from build123d import *

# Parameters (mm, degrees)
BOSS_EXTRUDE1_DEPTH = 29.765625
SKETCH3_R           = 29.464
OLEOPIST_DEPTH      = 397.764
SKETCH5_R           = 32.004
REFMAXOLEO_DEPTH    = 2.54
SKETCH7_R           = 9.525
BOSS_EXTRUDE4_DEPTH = 15.875


with BuildPart() as part:
    # Sketch1 → Boss-Extrude1 (new, symmetric)
    with BuildSketch(Plane.XY):
        with BuildLine():
            Line((-114.3, -150.1775), (-114.3, 150.1775))
            ThreePointArc((-114.3, 150.1775), (-99.421024484, 186.098524484), (-63.5, 200.9775))
            Line((-63.5, 200.9775), (15.875, 200.9775))
            Line((15.875, 200.9775), (15.875, 251.7775))
            Line((15.875, 251.7775), (-63.5, 251.7775))
            ThreePointArc((-63.5, 251.7775), (-135.342048969, 222.019548969), (-165.1, 150.1775))
            Line((-165.1, 150.1775), (-165.1, -150.1775))
            Line((-165.1, -150.1775), (-114.3, -150.1775))
        make_face()
    extrude(amount=BOSS_EXTRUDE1_DEPTH, both=True)

    # Sketch2 → Revolve1 (revolve)
    with BuildSketch(Plane.XZ.offset(150.1775)):
        Polygon((-165.1, 0), (-114.3, 0), (-50.8, 0), (-50.8, 81.915), (-76.2, 81.915), (-76.2, 31.75), (-114.3, 31.75), (-114.3, 37.20703125), (-165.1, 37.20703125), align=None)
    revolve(axis=Axis((-165.1, -150.1775, 0), (1, 0, 0)))

    # Sketch3 → OleoPist (add)
    with BuildSketch(Plane.XZ.offset(-200.9775)):
        with Locations(Location((15.875, 0, 0), (0, 0, 237.398482094))):
            Circle(SKETCH3_R)
    extrude(amount=-OLEOPIST_DEPTH)

    # Sketch5 → RefMaxOleo (add)
    with BuildSketch(Plane(origin=(0, 340.6775, 0), x_dir=(1, 0, 0), z_dir=(0, 1, 0))):
        with Locations(Location((15.875, 0, 0), (0, 0, 180))):
            Circle(SKETCH5_R)
    extrude(amount=-REFMAXOLEO_DEPTH)

    # Sketch7 → Boss-Extrude4 (add, symmetric)
    with BuildSketch(Plane(origin=(15.875, -150.1775, 0), x_dir=(0, 0, -1), z_dir=(1, 0, 0))):
        with BuildLine():
            Line((16.764, 488.315), (59.880363403, 435.864541166))
            ThreePointArc((59.880363403, 435.864541166), (65.58043358, 421.731246842), (62.165446707, 406.879355611))
            Line((62.165446707, 406.879355611), (29.464, 351.155))
            Line((29.464, 351.155), (16.764, 351.155))
            Line((16.764, 351.155), (16.764, 488.315))
        make_face()
        with Locations((40.259, 419.735)):
            Circle(SKETCH7_R, mode=Mode.SUBTRACT)
    extrude(amount=BOSS_EXTRUDE4_DEPTH, both=True)


solid = part.part
Source: CAD feature listing. Evaluate the final solid. Frame: model axes, mm. A direction names the side the tool comes from. Round coordinates to 2 decimals unless told otherwise and drop trailing zeros. Write each loop counter-clockwise with the first axis right and the second up, starting at its lowest first coordinate (ties: lowest second). Pieces come first, ordered by that corner, then holes. Notation, with made-up numbers: (52.5, 83.5) - (86.5, 83.5) arc R7 ccw to (86.5, 91.5) - close; hole circle Ø4 at (37, -7). An arc over 180 degrees is marked (long way). Use CSV: the item, a comma, the result in double quotes. Start each with the question number.
(1) Mould query, pull axis Z, two halves, no side actions, for faces 1 (the face through (-95.517, -181.657, -4.133)), 2 (the face through (6.5, 340.678, -28.3)), 3 (the face through (16, 279, -39)). Classes: pulls with the +Z half, pulls with the -Z half, needs draft (parallel to the pull), parting line crosses it, or undercut.
(2) Cut plane B-B, the plane y = -161. Return loops of the section in (x, z), and give its area (3 significant figures).
(3) First-contact query: pin 1 Ø6 at (x, z) = (-24.5, 3.5) entering from +Y; pin 2 Ø10 at (y, z) = (-4.5, -26) entering from +X; pin 3 Ø1 at (y, z) = (507, -7.5) entering from +X. Flat tips, straight axial feed; report the tip coordinate or a pass-through.
(4) Cut plane A-A, the plane z = 0. Return loops of the section in (x, y), and give its area (3 significant figures).
(5) Set-up query: faces 4 (the face through (-50.8, -151, 1)), 5 (the face through (42.55, 467.9, -12.51)), 6 (the face through (6.5, 338.138, -28.3)). Return all of +Z, -Z, +X, -X, +Y, -Y with unobstructed straight access to the full face (end or side cutting, diameter ignored); none if empty.
(6) Cut plane C-C, the plane x = -134. Return loops of the section in (y, z), and give its area (3 significant figures).
(7) Cut plane D-D, the plane y = 365.5. Return loops of the section in (x, z) (3 decimals).
(8) Material intervals for probe 1 along X at (y, z) = (-118.5, 24); probe 2 along Y at (x, z) = (-12, -8); probe 3 along X at (y, z) = (-139, 62.5), sorted ascending. Write a range as [from, to].
Geometry says:
1,face 1,"parting line crosses it"
1,face 2,"needs draft"
1,face 3,"undercut"
2,outline,"(-165.1, -35.6) - (-114.3, -35.6) - (-114.3, -29.85) - (-76.2, -29.85) - (-76.2, -81.2) - (-50.8, -81.2) - (-50.8, 81.2) - (-76.2, 81.2) - (-76.2, 29.85) - (-114.3, 29.85) - (-114.3, 35.6) - (-165.1, 35.6) - close"
2,area,"10,000 mm²"
3,pin 1,"y = 251.78"
3,pin 2,"x = -114.3"
3,pin 3,"x = 44.5"
4,outline,"(-165.1, -187.38) - (-114.3, -187.38) - (-114.3, -181.93) - (-76.2, -181.93) - (-76.2, -232.09) - (-50.8, -232.09) - (-50.8, -68.26) - (-76.2, -68.26) - (-76.2, -118.43) - (-114.3, -118.43) - (-114.3, 150.18) arc R50.8 cw to (-63.5, 200.98) - (45.34, 200.98) - (45.34, 338.14) - (47.88, 338.14) - (47.88, 340.68) - (45.34, 340.68) - (45.34, 598.74) - (-13.59, 598.74) - (-13.59, 340.68) - (-16.13, 340.68) - (-16.13, 338.14) - (-13.59, 338.14) - (-13.59, 251.78) - (-63.5, 251.78) arc R101.6 ccw to (-165.1, 150.18) - close"
4,area,"55,800 mm²"
5,face 4,"+Z, -Z, +X, -Y"
5,face 5,"+Y"
5,face 6,"none"
6,outline,"(-127.85, -29.77) - (223.34, -29.77) - (223.34, 29.77) - (-127.85, 29.77) arc R37.21 ccw (long way) to start"
6,area,"24,600 mm²"
7,outline,"circle Ø58.928 at (15.875, 0)"
8,probe 1,"[-165.1, -114.3], [-76.2, -50.8]"
8,probe 2,"[200.98, 598.74]"
8,probe 3,"[-76.2, -50.8]"
